```python
from build123d import *

# Parameters (mm, degrees)
BOSS_EXTRUDE1_DEPTH = 3.5


with BuildPart() as part:
    # Sketch1 → Boss-Extrude1 (new body)
    with BuildSketch(Plane(origin=(0, 0, 0), x_dir=(1, 0, 0), z_dir=(0, 1, 0))):
        with BuildLine():
            Line((-27.5, 32.5), (27.5, 32.5))
            ThreePointArc((27.5, 32.5), (31.035533906, 31.035533906), (32.5, 27.5))
            Line((32.5, 27.5), (32.5, -27.5))
            ThreePointArc((32.5, -27.5), (31.035533906, -31.035533906), (27.5, -32.5))
            Line((27.5, -32.5), (-27.5, -32.5))
            ThreePointArc((-27.5, -32.5), (-31.035533906, -31.035533906), (-32.5, -27.5))
            Line((-32.5, -27.5), (-32.5, 27.5))
            ThreePointArc((-32.5, 27.5), (-31.035533906, 31.035533906), (-27.5, 32.5))
        make_face()
        with BuildLine():
            Line((-21.5, -24.4), (-14.9, -24.4))
            ThreePointArc((-14.9, -24.4), (-13.4, -25.9), (-14.9, -27.4))
            Line((-14.9, -27.4), (-21.5, -27.4))
            ThreePointArc((-21.5, -27.4), (-23, -25.9), (-21.5, -24.4))
        make_face(mode=Mode.SUBTRACT)
        with BuildLine():
            Line((21.5, -27.4), (14.9, -27.4))
            ThreePointArc((14.9, -27.4), (13.4, -25.9), (14.9, -24.4))
            Line((14.9, -24.4), (21.5, -24.4))
            ThreePointArc((21.5, -24.4), (23, -25.9), (21.5, -27.4))
        make_face(mode=Mode.SUBTRACT)
        with BuildLine():
            Line((21.5, 24.4), (14.9, 24.4))
            ThreePointArc((14.9, 24.4), (13.4, 25.9), (14.9, 27.4))
            Line((14.9, 27.4), (21.5, 27.4))
            ThreePointArc((21.5, 27.4), (23, 25.9), (21.5, 24.4))
        make_face(mode=Mode.SUBTRACT)
        with BuildLine():
            Line((-21.5, 27.4), (-14.9, 27.4))
            ThreePointArc((-14.9, 27.4), (-13.4, 25.9), (-14.9, 24.4))
            Line((-14.9, 24.4), (-21.5, 24.4))
            ThreePointArc((-21.5, 24.4), (-23, 25.9), (-21.5, 27.4))
        make_face(mode=Mode.SUBTRACT)
        with BuildLine():
            Line((-3.3, -24.4), (3.3, -24.4))
            ThreePointArc((3.3, -24.4), (4.8, -25.9), (3.3, -27.4))
            Line((3.3, -27.4), (-3.3, -27.4))
            ThreePointArc((-3.3, -27.4), (-4.8, -25.9), (-3.3, -24.4))
        make_face(mode=Mode.SUBTRACT)
        with BuildLine():
            Line((-3.3, 27.4), (3.3, 27.4))
            ThreePointArc((3.3, 27.4), (4.8, 25.9), (3.3, 24.4))
            Line((3.3, 24.4), (-3.3, 24.4))
            ThreePointArc((-3.3, 24.4), (-4.8, 25.9), (-3.3, 27.4))
        make_face(mode=Mode.SUBTRACT)
    extrude(amount=BOSS_EXTRUDE1_DEPTH)


solid = part.part
```
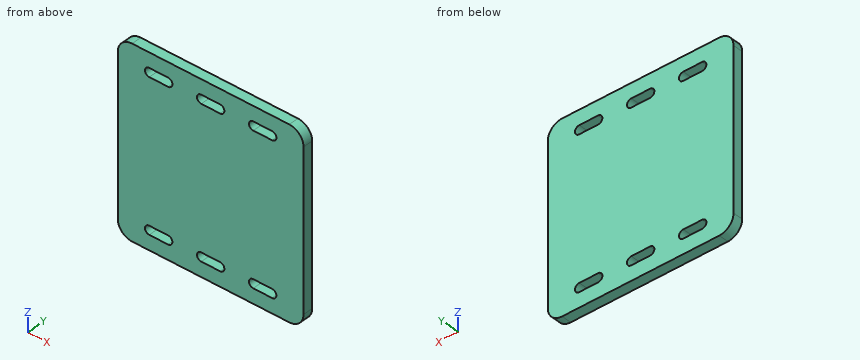
For this review, take the finished solid that the model builds, in its own axes (mm). Coordinates: 2 decimals unless noted, no trailing zeros. Write each loop counter-clockwise with the first axis right and the second up, starting at its lowest first coordinate (ties: lowest second). Pieces come first, ordered by that corner, then holes. Notation, with made-up numbers: (3.5, 63.25) -> (54.5, 63.25) arc R12 ccw to (54.5, 76.25) -> close; hole circle Ø4 at (21, -14). An arc over 180 degrees is marked (long way). Put each result on its own line as item: value.
Q1. Take a section at B-B, the plane y = 2.7. Count the separate pieces of the cut face and the enclosed holes in it, then the cut area to 3 significant figures.
From the geometry:
separate pieces: 1
enclosed holes: 6
area: 4,040 mm2
Q2. Take a section at C-C, the plane x = -20. State the section outline as (y, z) points.
From the geometry:
outline: (0, -32.5) -> (3.5, -32.5) -> (3.5, -27.4) -> (0, -27.4) -> close; (0, -24.4) -> (3.5, -24.4) -> (3.5, 24.4) -> (0, 24.4) -> close; (0, 27.4) -> (3.5, 27.4) -> (3.5, 32.5) -> (0, 32.5) -> close
Q3. Wall thickness on L1, parallel to Z at x = -15, y = 0.25; L2, parallel to X at y = 2.35, z = 29: over which ranges is each line inside the solid? List them lowest first.
From the geometry:
L1: z = -32.5 to -27.4, -24.4 to 24.4, 27.4 to 32.5
L2: x = -32.27 to 32.27
Q4. Take a section at A-A, the plane z = 25.9. State the section outline as (x, y) points, then the cut area to 3 significant figures.
From the geometry:
outline: (-32.5, 0) -> (-23, 0) -> (-23, 3.5) -> (-32.5, 3.5) -> close; (-13.4, 0) -> (-4.8, 0) -> (-4.8, 3.5) -> (-13.4, 3.5) -> close; (4.8, 0) -> (13.4, 0) -> (13.4, 3.5) -> (4.8, 3.5) -> close; (23, 0) -> (32.5, 0) -> (32.5, 3.5) -> (23, 3.5) -> close
area: 127 mm2
